```python
from build123d import *

# Parameters (mm, degrees)
BOSS_EXTRUDE1_DEPTH = 514.35
CUT_EXTRUDE1_REACH  = 516.35
SKETCH2_R           = 2.54


with BuildPart() as part:
    # Sketch1 → Boss-Extrude1 (new body)
    with BuildSketch(Plane(origin=(0, 0, 0), x_dir=(0, 0, -1), z_dir=(1, 0, 0))):
        Polygon((-3.666174209, 6.35), (0, 4.699060448), (3.666174209, 6.35), (4.069505722, 2.349530224), (7.332348419, 0), (4.069505722, -2.349530224), (3.666174209, -6.35), (0, -4.699060448), (-3.666174209, -6.35), (-4.069505722, -2.349530224), (-7.332348419, 0), (-4.069505722, 2.349530224), align=None)
    extrude(amount=BOSS_EXTRUDE1_DEPTH)

    # Sketch2 → Cut-Extrude1 (cut, up to next)
    with BuildSketch(Plane(origin=(514.35, 0, 0), x_dir=(0, 0, -1), z_dir=(1, 0, 0)), mode=Mode.PRIVATE) as cut_extrude1_sk1:
        Circle(SKETCH2_R)
    cut_extrude1_tool1 = extrude(cut_extrude1_sk1.sketch, amount=-CUT_EXTRUDE1_REACH, mode=Mode.PRIVATE) & part.part
    add(cut_extrude1_tool1.solids().sort_by_distance((514.35, 0, 0))[0], mode=Mode.SUBTRACT)


solid = part.part
```
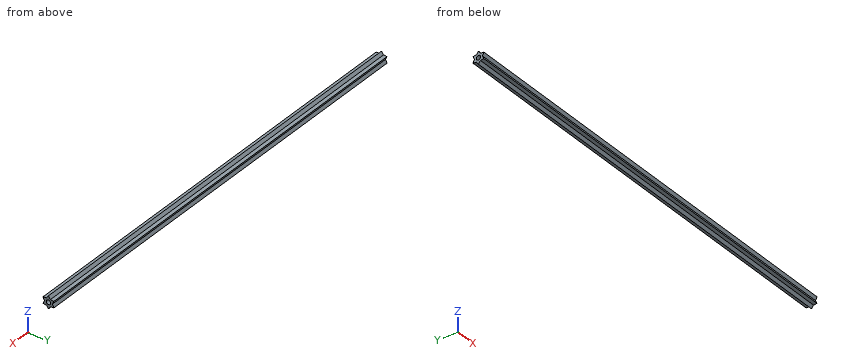
Verification items for the finished model (mm, model axes). Give positions to 0.01 mm unless a question says otherwise; leave off trailing zeros. Loops run counter-clockwise (first coordinate to the right, second up) from the corner with the lowest first, then second, coordinate; pieces in that order, holes last. Notation, with made-up numbers: M 13.25,25 L 35.25,25 A10 cw 35.25,30 Z; hole C -16.5,89.5 d11. An arc over 180 degrees is marked long. Return JSON: item names as keys, results as strings.
1) Gauge pin test, flat ends, axial feed: P1, Ø1, axis at x = 296.5, z = -2, coming from the -Y side; P2, Ø1, axis at x = 324, y = 1, coming from the +Z side; P3, Ø1.5, axis at x = 198, y = 2.5, coming from the +Z side. Record the tip position at first contact, or that the pin passes through.
Findings:
{"P1": "stops at y = -5.82", "P2": "stops at z = 6.64", "P3": "stops at z = 4.9"}
2) Section check A-A, the plane x = 81. Enter the section's corners in (y, z).
Findings:
{"outline": "M -6.35,-3.67 L -2.35,-4.07 L 0,-7.33 L 2.35,-4.07 L 6.35,-3.67 L 4.7,0 L 6.35,3.67 L 2.35,4.07 L 0,7.33 L -2.35,4.07 L -6.35,3.67 L -4.7,0 Z; hole C 0,0 d5.08"}
3) Material ranges on L1, parallel to Y at x = 344, z = 0; L2, parallel to Z at x = 207.5, y = -0.25; L3, parallel to Z at x = 186, y = 2, recorded low to high. Write a range as [from, to].
Findings:
{"L1": "y = [-4.7, -2.54], [2.54, 4.7]", "L2": "z = [-6.99, -2.53], [2.53, 6.99]", "L3": "z = [-4.55, -1.57], [1.57, 4.55]"}
